Part print with two shaded views. Sizes in mm from the minimum x, y, z corner. Give positions to 0.01 mm unless a question says otherwise; leave off trailing zeros. Loops run counter-clockwise (first coordinate to the right, second up) from the corner with the lowest first, then second, coordinate; pieces in that order, holes last. Notation, with made-up numbers: M -20.5,9 L 16.5,9 A17 cw 16.5,24 Z; hole C 74.5,24.25 d5. An arc over 180 degrees is marked long. Answer in a Markdown table with one row per item.
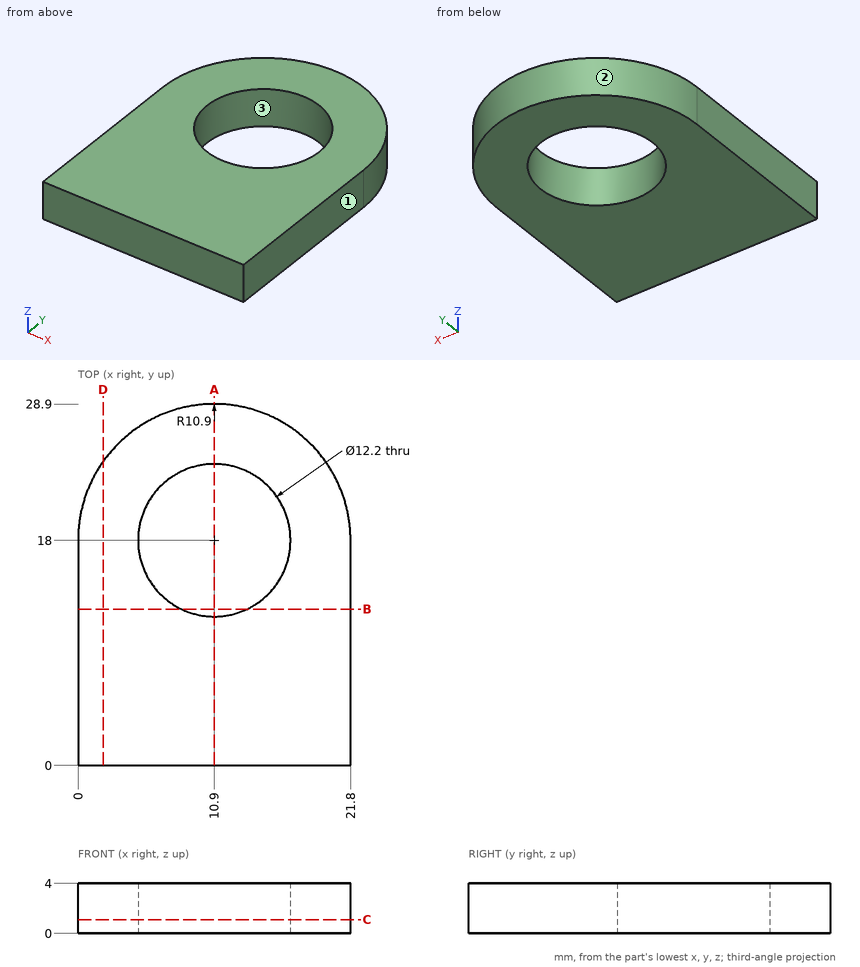
Q1. Probe probe 1 along Y at (x, z) = (10.9, 1.8); probe 2 along Y at (x, z) = (7.25, 1.15); probe 3 along X at (y, z) = (19.5, 1.6). List the from-to ranges inside material, lowest first.
Reported:
| item | result |
|---|---|
| probe 1 | 0 to 11.9, 24.1 to 28.9 |
| probe 2 | 0 to 13.11, 22.89 to 28.27 |
| probe 3 | 0.1 to 4.99, 16.81 to 21.7 |
Q2. Saw through at D-D (x = 2). Give the cut face in (y, z).
Reported:
| item | result |
|---|---|
| outline | M 0,0 L 24.29,0 L 24.29,4 L 0,4 Z |
Q3. Saw through at C-C (z = 1.1). Give the cut face in (x, y), and give its area (3 significant figures).
Reported:
| item | result |
|---|---|
| outline | M 0,0 L 21.8,0 L 21.8,18 A10.9 ccw 0,18 Z; hole C 10.9,18 d12.2 |
| area | 462 mm² |
Q4. Mould opens along Y. For the marked faces 1, 2 and 3 say: released by +Y, released by -Y, zero draft, split by the parting line, or undercut.
Reported:
| item | result |
|---|---|
| face 1 | zero draft |
| face 2 | released by +Y |
| face 3 | undercut |
Q5. Drop a flat-ended pin along its axis: pin 1 (7.5 mm diameter, centred on x = 10.9, y = 18, fed in from +Z). Give the stop position or say it passes through.
Reported:
| item | result |
|---|---|
| pin 1 | through |
Q6. Saw through at B-B (y = 12.5). Give the cut face in (x, z), and give its area (3 significant figures).
Reported:
| item | result |
|---|---|
| outline | M 0,0 L 8.26,0 L 8.26,4 L 0,4 Z; M 13.54,0 L 21.8,0 L 21.8,4 L 13.54,4 Z |
| area | 66.1 mm² |
Q7. Saw through at A-A (x = 10.9). Give the cut face in (y, z), and give its area (3 significant figures).
Reported:
| item | result |
|---|---|
| outline | M 0,0 L 11.9,0 L 11.9,4 L 0,4 Z; M 24.1,0 L 28.9,0 L 28.9,4 L 24.1,4 Z |
| area | 66.8 mm² |
